```python
from build123d import *

# Parameters (mm, degrees)
SKETCH1_R           = 3.55
SKETCH1_R_2         = 2.6
BOSS_EXTRUDE1_DEPTH = 3


with BuildPart() as part:
    # Sketch1 → Boss-Extrude1 (new body)
    with BuildSketch(Plane(origin=(0, 0, 0), x_dir=(1, 0, 0), z_dir=(0, 1, 0))):
        with BuildLine():
            Line((40, -60), (-40, -60))
            ThreePointArc((-40, -60), (-47.071067812, -57.071067812), (-50, -50))
            Line((-50, -50), (-50, 50))
            ThreePointArc((-50, 50), (-47.071067812, 57.071067812), (-40, 60))
            Line((-40, 60), (40, 60))
            ThreePointArc((40, 60), (47.071067812, 57.071067812), (50, 50))
            Line((50, 50), (50, -50))
            ThreePointArc((50, -50), (47.071067812, -57.071067812), (40, -60))
        make_face()
        with Locations((-22.3, 42.3)):
            Circle(SKETCH1_R, mode=Mode.SUBTRACT)
        with Locations((0, 10)):
            Circle(SKETCH1_R_2, mode=Mode.SUBTRACT)
        Circle(SKETCH1_R_2, mode=Mode.SUBTRACT)
        with Locations((10, 0)):
            Circle(SKETCH1_R_2, mode=Mode.SUBTRACT)
        with Locations((-10, 0)):
            Circle(SKETCH1_R_2, mode=Mode.SUBTRACT)
        with Locations((-32.3, 42.3)):
            Circle(SKETCH1_R, mode=Mode.SUBTRACT)
        with Locations((-32.3, 0)):
            Circle(SKETCH1_R, mode=Mode.SUBTRACT)
        with Locations((-32.3, -42.3)):
            Circle(SKETCH1_R, mode=Mode.SUBTRACT)
        with Locations((-20, 10)):
            Circle(SKETCH1_R_2, mode=Mode.SUBTRACT)
        with Locations((-40, 10)):
            Circle(SKETCH1_R_2, mode=Mode.SUBTRACT)
        with Locations((-10, 20)):
            Circle(SKETCH1_R_2, mode=Mode.SUBTRACT)
        with Locations((-10, 30)):
            Circle(SKETCH1_R_2, mode=Mode.SUBTRACT)
        with Locations((-10, 42.3)):
            Circle(SKETCH1_R_2, mode=Mode.SUBTRACT)
        with Locations((0, 42.3)):
            Circle(SKETCH1_R_2, mode=Mode.SUBTRACT)
        with Locations((10, 42.3)):
            Circle(SKETCH1_R_2, mode=Mode.SUBTRACT)
        with Locations((10, 30)):
            Circle(SKETCH1_R_2, mode=Mode.SUBTRACT)
        with Locations((10, 20)):
            Circle(SKETCH1_R_2, mode=Mode.SUBTRACT)
        with Locations((20, 10)):
            Circle(SKETCH1_R_2, mode=Mode.SUBTRACT)
        with Locations((40, 10)):
            Circle(SKETCH1_R_2, mode=Mode.SUBTRACT)
        with Locations((22.3, 42.3)):
            Circle(SKETCH1_R_2, mode=Mode.SUBTRACT)
        with Locations((32.3, 42.3)):
            Circle(SKETCH1_R_2, mode=Mode.SUBTRACT)
        with Locations((32.3, 0)):
            Circle(SKETCH1_R_2, mode=Mode.SUBTRACT)
        with Locations((40, -10)):
            Circle(SKETCH1_R_2, mode=Mode.SUBTRACT)
        with Locations((32.3, -42.3)):
            Circle(SKETCH1_R_2, mode=Mode.SUBTRACT)
        with Locations((22.3, -42.3)):
            Circle(SKETCH1_R_2, mode=Mode.SUBTRACT)
        with Locations((20, -10)):
            Circle(SKETCH1_R_2, mode=Mode.SUBTRACT)
        with Locations((0, -10)):
            Circle(SKETCH1_R_2, mode=Mode.SUBTRACT)
        with Locations((10, -20)):
            Circle(SKETCH1_R_2, mode=Mode.SUBTRACT)
        with Locations((10, -30)):
            Circle(SKETCH1_R_2, mode=Mode.SUBTRACT)
        with Locations((10, -42.3)):
            Circle(SKETCH1_R_2, mode=Mode.SUBTRACT)
        with Locations((0, -42.3)):
            Circle(SKETCH1_R_2, mode=Mode.SUBTRACT)
        with Locations((-10, -42.3)):
            Circle(SKETCH1_R_2, mode=Mode.SUBTRACT)
        with Locations((-10, -30)):
            Circle(SKETCH1_R_2, mode=Mode.SUBTRACT)
        with Locations((-10, -20)):
            Circle(SKETCH1_R_2, mode=Mode.SUBTRACT)
        with Locations((-20, -10)):
            Circle(SKETCH1_R_2, mode=Mode.SUBTRACT)
        with Locations((-40, -10)):
            Circle(SKETCH1_R_2, mode=Mode.SUBTRACT)
        with Locations((-22.3, -42.3)):
            Circle(SKETCH1_R, mode=Mode.SUBTRACT)
    extrude(amount=BOSS_EXTRUDE1_DEPTH)


solid = part.part
```
Source: CAD feature listing. Evaluate the final solid. Frame: model axes, mm. Give positions to 0.01 mm unless a question says otherwise; leave off trailing zeros. Order: outer loops, then holes, each group sorted by start corner. A loop starts at its lowest first (then second) coordinate and runs counter-clockwise, first axis right, second up. Notation, with made-up numbers: (60, -27) -> (112, -27) arc R22 ccw to (112, -8) -> close; hole circle Ø10 at (69, 36.5). An arc over 180 degrees is marked (long way). Use a Markdown table: item, result.
Q1. Section C-C (z = -42.3). State how many separate pieces and enclosed holes the cut face has, and give its area (3 significant figures).
A:
| item | result |
|---|---|
| separate pieces | 8 |
| enclosed holes | 0 |
| area | 179 mm^2 |
Q2. Section B-B (x = 1). Return the cut outline in (y, z).
A:
| item | result |
|---|---|
| outline | (0, -60) -> (3, -60) -> (3, -44.7) -> (0, -44.7) -> close; (0, -39.9) -> (3, -39.9) -> (3, -12.4) -> (0, -12.4) -> close; (0, -7.6) -> (3, -7.6) -> (3, -2.4) -> (0, -2.4) -> close; (0, 2.4) -> (3, 2.4) -> (3, 7.6) -> (0, 7.6) -> close; (0, 12.4) -> (3, 12.4) -> (3, 39.9) -> (0, 39.9) -> close; (0, 44.7) -> (3, 44.7) -> (3, 60) -> (0, 60) -> close |
Q3. Material intervals for line 1 (X direction, y = 2.1, z = 0); line 2 (X direction, y = 2.3, z = 20); line 3 (X direction, y = 2.25, z = 10), sorted ascending. Write a range as [from, to].
A:
| item | result |
|---|---|
| line 1 | [-50, -35.85], [-28.75, -12.6], [-7.4, -2.6], [2.6, 7.4], [12.6, 29.7], [34.9, 50] |
| line 2 | [-50, -12.6], [-7.4, 7.4], [12.6, 50] |
| line 3 | [-50, -42.6], [-37.4, -22.6], [-17.4, -2.6], [2.6, 17.4], [22.6, 37.4], [42.6, 50] |
Q4. Section D-D (x = 32.3). Return the cut outline in (y, z), and give its area (3 significant figures).
A:
| item | result |
|---|---|
| outline | (0, -60) -> (3, -60) -> (3, -44.9) -> (0, -44.9) -> close; (0, -39.7) -> (3, -39.7) -> (3, -2.6) -> (0, -2.6) -> close; (0, 2.6) -> (3, 2.6) -> (3, 39.7) -> (0, 39.7) -> close; (0, 44.9) -> (3, 44.9) -> (3, 60) -> (0, 60) -> close |
| area | 313 mm^2 |
Q5. Section A-A (z = 0). Return the cut outline in (x, y).
A:
| item | result |
|---|---|
| outline | (-50, 0) -> (-35.85, 0) -> (-35.85, 3) -> (-50, 3) -> close; (-28.75, 0) -> (-12.6, 0) -> (-12.6, 3) -> (-28.75, 3) -> close; (-7.4, 0) -> (-2.6, 0) -> (-2.6, 3) -> (-7.4, 3) -> close; (2.6, 0) -> (7.4, 0) -> (7.4, 3) -> (2.6, 3) -> close; (12.6, 0) -> (29.7, 0) -> (29.7, 3) -> (12.6, 3) -> close; (34.9, 0) -> (50, 0) -> (50, 3) -> (34.9, 3) -> close |
Q6. Pull-direction query (X, two-part tool) for faces 1 (the face through (12, 3, 12)), 2 (the face through (-28.914, 1.479, 41.234)), 3 (the face through (50, 1, -1)); classes: +X half, -X half, draft (parallel to the pull), parting line (faces both ways), or undercut.
A:
| item | result |
|---|---|
| face 1 | draft |
| face 2 | undercut |
| face 3 | +X half |
